Could you check a few things on this model? Use its own coordinates, in mm. Give positions to 0.01 mm unless a question says otherwise; leave off trailing zeros. Loops run counter-clockwise (first coordinate to the right, second up) from the corner with the lowest first, then second, coordinate; pieces in that order, holes last.
1. Imagine slicing it at B-B (x = -16.5). List the corners of the cut face in (y, z) for me.
2. For P1, Ø3, axis at y = -2.5, z = 15, coming from the +X side; P2, Ø5, axis at x = -17.5, y = -0.5, coming from the -Z side, each with a flat end and sliding along its axis, tell me the tip position at first contact or that it passes through.
3. I need wall thicknesses on line 1 along Y through (x, z) = (-13.75, 20.5); line 2 along Z through (x, y) = (-18.5, 1.75); line 3 along X through (y, z) = (-1.75, 13). Which ranges of each line are inside material? Lowest first, please.
4. Imagine slicing it at D-D (x = -7.25). List the corners of the cut face in (y, z) for me, plus the area to 3 significant figures.
5. Thinking about a two-plate mould opening in Z: for faces 1 (the flat face through (-18, -8.642, 12)), 2 (the flat face through (-15, 9, 5.839)), 3 (the flat face through (-15, 9, 23.839)), 4 (the cylindrical face through (-16.13, -2.56, 9.63)), which applies, +Z half, -Z half, draft (parallel to the pull), parting line (faces both ways), or undercut?
6. Imagine slicing it at C-C (y = -5.25). List the corners of the cut face in (x, z) for me, plus the area to 3 significant figures.
7. Imagine slicing it at A-A (z = 9.5). List the corners of the cut face in (x, y) for me.
```python
from build123d import *

# Parameters (mm, degrees)
ESQUISSE1_W         = 30
ESQUISSE1_H         = 20
BOSS_EXTRU_1_DEPTH  = 30
SKETCH1_R           = 5
BOSS_EXTRUDE1_DEPTH = 20
SCALE1_SCALE        = 0.6


with BuildPart() as part:
    # Esquisse1 → Boss.-Extru.1 (new body)
    with BuildSketch(Plane.XY):
        with Locations((-15, 10)):
            Rectangle(ESQUISSE1_W, ESQUISSE1_H)
    extrude(amount=BOSS_EXTRU_1_DEPTH)

    # Sketch1 → Boss-Extrude1 (add)
    with BuildSketch(Plane(origin=(0, 0, 0), x_dir=(1, 0, 0), z_dir=(0, 1, 0))):
        with Locations(Location((-20, -10, 0), (0, 0, 270))):
            Circle(SKETCH1_R)
    extrude(amount=-BOSS_EXTRUDE1_DEPTH)


with BuildPart() as part_1:
    # Scale1: scaled about (-15.401311296, 8.394754817, 14.598688704)
    add(part.part.scale(SCALE1_SCALE).moved(Location((-6.160524518, 3.357901927, 5.839475482))))


solid = part_1.part
```
Derived:
1. outline: (-8.64, 9.34) - (3.36, 9.34) - (3.36, 5.84) - (15.36, 5.84) - (15.36, 23.84) - (3.36, 23.84) - (3.36, 14.34) - (-8.64, 14.34) - close
2. P1: stops at x = -15.66
2. P2: stops at z = 8.84
3. line 1: y = 3.36 to 15.36
3. line 2: z = 8.86 to 14.82
3. line 3: x = -20.93 to -15.39
4. outline: (3.36, 5.84) - (15.36, 5.84) - (15.36, 23.84) - (3.36, 23.84) - close
4. area: 216 mm2
5. face 1: draft
5. face 2: -Z half
5. face 3: +Z half
5. face 4: parting line
6. outline: circle Ø6 at (-18.16, 11.84)
6. area: 28.3 mm2
7. outline: (-24.16, 3.36) - (-20.04, 3.36) - (-20.04, -8.64) - (-16.28, -8.64) - (-16.28, 3.36) - (-6.16, 3.36) - (-6.16, 15.36) - (-24.16, 15.36) - close
